from build123d import *

# Parameters (mm, degrees)
SKETCH1_W           = 55
SKETCH1_H           = 85
SKETCH1_R           = 2.75
SKETCH1_R_2         = 3.5
BOSS_EXTRUDE1_DEPTH = 5


with BuildPart() as part:
    # Sketch1 → Boss-Extrude1 (new body)
    with BuildSketch(Plane.XZ):
        with Locations((7.5, 0)):
            Rectangle(SKETCH1_W, SKETCH1_H)
        with Locations(Location((14, 10.5, 0), (0, 0, 90))):
            Circle(SKETCH1_R, mode=Mode.SUBTRACT)
        with Locations(Location((-14, 10.5, 0), (0, 0, 90))):
            Circle(SKETCH1_R, mode=Mode.SUBTRACT)
        with Locations(Location((-14, -10.5, 0), (0, 0, 90))):
            Circle(SKETCH1_R, mode=Mode.SUBTRACT)
        with Locations(Location((14, -10.5, 0), (0, 0, 90))):
            Circle(SKETCH1_R, mode=Mode.SUBTRACT)
        with Locations(Location((28, 37.5, 0), (0, 0, 90))):
            Circle(SKETCH1_R, mode=Mode.SUBTRACT)
        with Locations(Location((28, 5.5, 0), (0, 0, 90))):
            Circle(SKETCH1_R, mode=Mode.SUBTRACT)
        with Locations(Location((28, -5.5, 0), (0, 0, 90))):
            Circle(SKETCH1_R, mode=Mode.SUBTRACT)
        with Locations(Location((28, -37.5, 0), (0, 0, 90))):
            Circle(SKETCH1_R, mode=Mode.SUBTRACT)
        with Locations(Location((0, 0, 0), (0, 0, 90))):
            Circle(SKETCH1_R_2, mode=Mode.SUBTRACT)
    extrude(amount=-BOSS_EXTRUDE1_DEPTH)


solid = part.part
Work out the finished part from the listing and answer in its coordinate system (mm). Give positions to 0.01 mm unless a question says otherwise; leave off trailing zeros. Write each loop counter-clockwise with the first axis right and the second up, starting at its lowest first coordinate (ties: lowest second). Pieces come first, ordered by that corner, then holes. Notation, with made-up numbers: (-17, 83) - (38, 83) arc R23 cw to (38, 103) - close; hole circle Ø7 at (58, 28). An arc over 180 degrees is marked (long way). One line per item, written item: value. Start each with the question number.
1. Given pin 1 (7 mm diameter, centred on x = 28, z = 5.5, fed in from -Y), flat-ended and moving along its own axis, determine where the tip first touches the part or whether it passes through.
2. Consider probe 1 along Z at (x, y) = (28, 3.4); probe 2 along Z at (x, y) = (14, 2.6); probe 3 along X at (y, z) = (3.4, 10.5). Determine where each line is inside the solid, lowest interval first.
3. Find section D-D (x = 0). Write down the section's boundary in (y, z), then the cut area to 3 significant figures.
4. Find section C-C (z = 10.5). Write down the section's boundary in (x, y).
5. For a pull along X with two mould halves and no side action, classify faces 1 (the flat face through (7, 2, 42.5)), 2 (the flat face through (-20, 2, -1)), 3 (the flat face through (35, 2, -1)), 4 (the cylindrical face through (-16.727, 2.465, 10.142)) as +X half, -X half, draft (parallel to the pull), parting line (faces both ways), or undercut.
6. Find section B-B (z = -5.5). Write down the section's boundary in (x, y).
7. Find section A-A (x = 28). Write down the section's boundary in (y, z), then the cut area to 3 significant figures.
Geometry results:
1. pin 1: y = 0
2. probe 1: -42.5 to -40.25, -34.75 to -8.25, -2.75 to 2.75, 8.25 to 34.75, 40.25 to 42.5
2. probe 2: -42.5 to -13.25, -7.75 to 7.75, 13.25 to 42.5
2. probe 3: -20 to -16.75, -11.25 to 11.25, 16.75 to 35
3. outline: (0, -42.5) - (5, -42.5) - (5, -3.5) - (0, -3.5) - close; (0, 3.5) - (5, 3.5) - (5, 42.5) - (0, 42.5) - close
3. area: 390 mm2
4. outline: (-20, 0) - (-16.75, 0) - (-16.75, 5) - (-20, 5) - close; (-11.25, 0) - (11.25, 0) - (11.25, 5) - (-11.25, 5) - close; (16.75, 0) - (35, 0) - (35, 5) - (16.75, 5) - close
5. face 1: draft
5. face 2: -X half
5. face 3: +X half
5. face 4: undercut
6. outline: (-20, 0) - (25.25, 0) - (25.25, 5) - (-20, 5) - close; (30.75, 0) - (35, 0) - (35, 5) - (30.75, 5) - close
7. outline: (0, -42.5) - (5, -42.5) - (5, -40.25) - (0, -40.25) - close; (0, -34.75) - (5, -34.75) - (5, -8.25) - (0, -8.25) - close; (0, -2.75) - (5, -2.75) - (5, 2.75) - (0, 2.75) - close; (0, 8.25) - (5, 8.25) - (5, 34.75) - (0, 34.75) - close; (0, 40.25) - (5, 40.25) - (5, 42.5) - (0, 42.5) - close
7. area: 315 mm2
